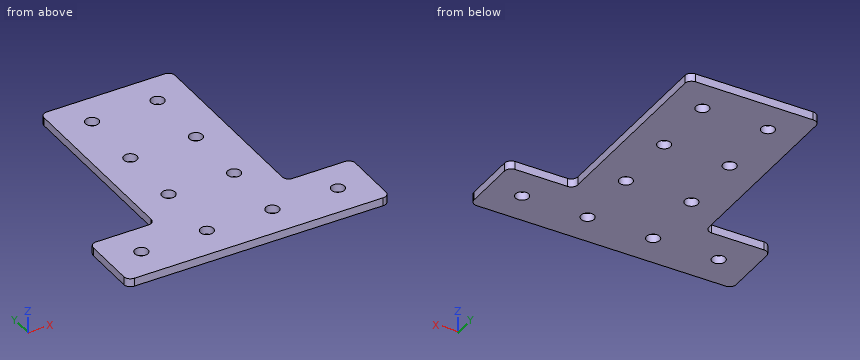
from build123d import *

# Parameters (mm, degrees)
BOSS_EXTRUDE1_DEPTH    = 3.175
FILLET1_R              = 2.54
F_10_CLEARANCE_HOLE1_D = 5.1054
F_10_CLEARANCE_HOLE2_D = 5.1054


with BuildPart() as part:
    # Sketch1 → Boss-Extrude1 (new body)
    with BuildSketch(Plane.XY):
        Polygon((-76.2, 25.4), (-101.6, 25.4), (-101.6, 0), (0, 0), (0, 25.4), (-25.4, 25.4), (-25.4, 101.6), (-76.2, 101.6), align=None)
    extrude(amount=BOSS_EXTRUDE1_DEPTH)

    # Fillet1
    fillet1_edges = [part.edges().sort_by_distance(p)[0] for p in [
        (0, 0, 1.5875),
        (-101.6, 0, 1.5875),
        (-101.6, 25.4, 1.5875),
        (-76.2, 25.4, 1.5875),
        (-76.2, 101.6, 1.5875),
        (-25.4, 101.6, 1.5875),
        (-25.4, 25.4, 1.5875),
        (0, 25.4, 1.5875),
    ]]
    fillet(fillet1_edges, radius=FILLET1_R)

    # #10 Clearance Hole1 (through all)
    with Locations(Plane.XY.offset(3.175)):
        with Locations((-63.5, 88.9), (-63.5, 63.5), (-63.5, 38.1), (-38.1, 88.9), (-38.1, 63.5), (-38.1, 38.1)):
            Hole(F_10_CLEARANCE_HOLE1_D / 2)

    # #10 Clearance Hole2 (through all)
    with Locations(Plane(origin=(0, 0, 0), x_dir=(1, 0, 0), z_dir=(0, 0, -1))):
        with Locations((-88.9, -12.7), (-63.5, -12.7), (-38.1, -12.7), (-12.7, -12.7)):
            Hole(F_10_CLEARANCE_HOLE2_D / 2)


solid = part.part
Geometry check sheet. Reference: the model listing, model coordinates, mm. Round coordinates to 2 decimals unless told otherwise and drop trailing zeros. Loops run counter-clockwise (first coordinate to the right, second up) from the corner with the lowest first, then second, coordinate; pieces in that order, holes last.
Item 1: Cross-section at B-B on z = 1.95. Count the separate pieces of the cut face and the enclosed holes in it, then the cut area to 3 significant figures.
Item 2: Thickness scan on line 1 (Y direction, x = -63.5, z = 0.8); line 2 (X direction, y = 89.5, z = 0.7); line 3 (Y direction, x = -37, z = 2.3). Record the ranges inside material, lowest first.
Item 3: Cross-section at D-D on y = 63.5. Record the boundary of the cut face in (x, z) (3 decimals), then the cut area to 3 significant figures.
Item 4: Gauge pin test, flat ends, axial feed: pin 1 (6 mm diameter, centred on x = -63.5, y = 88.9, fed in from +Z) (3 decimals); pin 2 (4 mm diameter, centred on x = -38.1, y = 88.9, fed in from +Z); pin 3 (1.6 mm diameter, centred on y = 75, z = 1, fed in from +X); pin 4 (1 mm diameter, centred on x = -12.5, z = 2.5, fed in from +Y). Record the tip position at first contact, or that the pin passes through.
Item 5: Cross-section at A-A on x = -12.7. Record the boundary of the cut face in (y, z) (3 decimals), then the cut area to 3 significant figures.
Item 6: Cross-section at C-C on x = -63.5. Record the boundary of the cut face in (y, z) (3 decimals), then the cut area to 3 significant figures.
Answer sheet:
1. separate pieces: 1
1. enclosed holes: 10
1. area: 6,240 mm2
2. line 1: y = 0 to 10.15, 15.25 to 35.55, 40.65 to 60.95, 66.05 to 86.35, 91.45 to 101.6
2. line 2: x = -76.2 to -65.98, -61.02 to -40.58, -35.62 to -25.4
2. line 3: y = 0 to 10.4, 15 to 35.8, 40.4 to 61.2, 65.8 to 86.6, 91.2 to 101.6
3. outline: (-76.2, 0) - (-66.053, 0) - (-66.053, 3.175) - (-76.2, 3.175) - close; (-60.947, 0) - (-40.653, 0) - (-40.653, 3.175) - (-60.947, 3.175) - close; (-35.547, 0) - (-25.4, 0) - (-25.4, 3.175) - (-35.547, 3.175) - close
3. area: 129 mm2
4. pin 1: stops at z = 3.175
4. pin 2: passes through
4. pin 3: stops at x = -25.4
4. pin 4: stops at y = 25.4
5. outline: (0, 0) - (10.147, 0) - (10.147, 3.175) - (0, 3.175) - close; (15.253, 0) - (25.4, 0) - (25.4, 3.175) - (15.253, 3.175) - close
5. area: 64.4 mm2
6. outline: (0, 0) - (10.147, 0) - (10.147, 3.175) - (0, 3.175) - close; (15.253, 0) - (35.547, 0) - (35.547, 3.175) - (15.253, 3.175) - close; (40.653, 0) - (60.947, 0) - (60.947, 3.175) - (40.653, 3.175) - close; (66.053, 0) - (86.347, 0) - (86.347, 3.175) - (66.053, 3.175) - close; (91.453, 0) - (101.6, 0) - (101.6, 3.175) - (91.453, 3.175) - close
6. area: 258 mm2
